```python
from build123d import *

# Parameters (mm, degrees)
EXTRUSION1_DEPTH         = 3
ENL_V_MAT_EXTRU_14_REACH = 176.1
ESQUISSE8_R              = 2
ESQUISSE10_R             = 2
ENL_V_MAT_EXTRU_16_DEPTH = 175.099861741
ENL_V_MAT_EXTRU_17_DEPTH = 175.099861741
ENL_V_MAT_EXTRU_18_DEPTH = 167.529952384
CONG_1_R                 = 3


with BuildPart() as part:
    # Esquisse1 → Extrusion1 (new body)
    with BuildSketch(Plane(origin=(0, 0, 0), x_dir=(1, 0, 0), z_dir=(0, 1, 0))):
        Polygon((-64.179491924, 79.940798285), (98.820508076, 79.940798285), (103.820508076, 74.940798285), (103.820508076, 24.940798285), (101.320508076, 15.610671266), (19.820508076, -125.551469551), (12.990381057, -127.38159657), (-30.310889132, -102.38159657), (-37.141016151, -95.551469551), (-118.641016151, 45.610671266), (-116.810889132, 52.440798285), (-73.509618943, 77.440798285), align=None)
    extrude(amount=EXTRUSION1_DEPTH)

    # Esquisse8 → Enlèv. mat.-Extru.14 (cut, up to next)
    with BuildSketch(Plane(origin=(0, 3, 0), x_dir=(1, 0, 0), z_dir=(0, 1, 0)), mode=Mode.PRIVATE) as enl_v_mat_extru_14_sk1:
        with Locations(Location((-100.570508076, 34.31163316, 0), (0, 0, 270))):
            Circle(ESQUISSE8_R)
    enl_v_mat_extru_14_tool1 = extrude(enl_v_mat_extru_14_sk1.sketch, amount=-ENL_V_MAT_EXTRU_14_REACH, mode=Mode.PRIVATE) & part.part
    # Esquisse8 → Enlèv. mat.-Extru.14 (cut, up to next)
    with BuildSketch(Plane(origin=(0, 3, 0), x_dir=(1, 0, 0), z_dir=(0, 1, 0)), mode=Mode.PRIVATE) as enl_v_mat_extru_14_sk2:
        with Locations(Location((80, 69.940798285, 0), (0, 0, 270))):
            Circle(ESQUISSE8_R)
    enl_v_mat_extru_14_tool2 = extrude(enl_v_mat_extru_14_sk2.sketch, amount=-ENL_V_MAT_EXTRU_14_REACH, mode=Mode.PRIVATE) & part.part
    # Esquisse8 → Enlèv. mat.-Extru.14 (cut, up to next)
    with BuildSketch(Plane(origin=(0, 3, 0), x_dir=(1, 0, 0), z_dir=(0, 1, 0)), mode=Mode.PRIVATE) as enl_v_mat_extru_14_sk3:
        with Locations(Location((50, 69.940798285, 0), (0, 0, 270))):
            Circle(ESQUISSE8_R)
    enl_v_mat_extru_14_tool3 = extrude(enl_v_mat_extru_14_sk3.sketch, amount=-ENL_V_MAT_EXTRU_14_REACH, mode=Mode.PRIVATE) & part.part
    # Esquisse8 → Enlèv. mat.-Extru.14 (cut, up to next)
    with BuildSketch(Plane(origin=(0, 3, 0), x_dir=(1, 0, 0), z_dir=(0, 1, 0)), mode=Mode.PRIVATE) as enl_v_mat_extru_14_sk4:
        with Locations(Location((-50.570508076, -52.290907218, 0), (0, 0, 270))):
            Circle(ESQUISSE8_R)
    enl_v_mat_extru_14_tool4 = extrude(enl_v_mat_extru_14_sk4.sketch, amount=-ENL_V_MAT_EXTRU_14_REACH, mode=Mode.PRIVATE) & part.part
    # Esquisse8 → Enlèv. mat.-Extru.14 (cut, up to next)
    with BuildSketch(Plane(origin=(0, 3, 0), x_dir=(1, 0, 0), z_dir=(0, 1, 0)), mode=Mode.PRIVATE) as enl_v_mat_extru_14_sk5:
        with Locations(Location((-35.570508076, -78.271669332, 0), (0, 0, 270))):
            Circle(ESQUISSE8_R)
    enl_v_mat_extru_14_tool5 = extrude(enl_v_mat_extru_14_sk5.sketch, amount=-ENL_V_MAT_EXTRU_14_REACH, mode=Mode.PRIVATE) & part.part
    # Esquisse8 → Enlèv. mat.-Extru.14 (cut, up to next)
    with BuildSketch(Plane(origin=(0, 3, 0), x_dir=(1, 0, 0), z_dir=(0, 1, 0)), mode=Mode.PRIVATE) as enl_v_mat_extru_14_sk6:
        with Locations(Location((-20, 69.940798285, 0), (0, 0, 270))):
            Circle(ESQUISSE8_R)
    enl_v_mat_extru_14_tool6 = extrude(enl_v_mat_extru_14_sk6.sketch, amount=-ENL_V_MAT_EXTRU_14_REACH, mode=Mode.PRIVATE) & part.part
    # Esquisse8 → Enlèv. mat.-Extru.14 (cut, up to next)
    with BuildSketch(Plane(origin=(0, 3, 0), x_dir=(1, 0, 0), z_dir=(0, 1, 0)), mode=Mode.PRIVATE) as enl_v_mat_extru_14_sk7:
        with Locations(Location((-50, 69.940798285, 0), (0, 0, 270))):
            Circle(ESQUISSE8_R)
    enl_v_mat_extru_14_tool7 = extrude(enl_v_mat_extru_14_sk7.sketch, amount=-ENL_V_MAT_EXTRU_14_REACH, mode=Mode.PRIVATE) & part.part
    # Esquisse8 → Enlèv. mat.-Extru.14 (cut, up to next)
    with BuildSketch(Plane(origin=(0, 3, 0), x_dir=(1, 0, 0), z_dir=(0, 1, 0)), mode=Mode.PRIVATE) as enl_v_mat_extru_14_sk8:
        with Locations(Location((20.570508076, -104.252431445, 0), (0, 0, 270))):
            Circle(ESQUISSE8_R)
    enl_v_mat_extru_14_tool8 = extrude(enl_v_mat_extru_14_sk8.sketch, amount=-ENL_V_MAT_EXTRU_14_REACH, mode=Mode.PRIVATE) & part.part
    # Esquisse8 → Enlèv. mat.-Extru.14 (cut, up to next)
    with BuildSketch(Plane(origin=(0, 3, 0), x_dir=(1, 0, 0), z_dir=(0, 1, 0)), mode=Mode.PRIVATE) as enl_v_mat_extru_14_sk9:
        with Locations(Location((35.570508076, -78.271669332, 0), (0, 0, 270))):
            Circle(ESQUISSE8_R)
    enl_v_mat_extru_14_tool9 = extrude(enl_v_mat_extru_14_sk9.sketch, amount=-ENL_V_MAT_EXTRU_14_REACH, mode=Mode.PRIVATE) & part.part
    # Esquisse8 → Enlèv. mat.-Extru.14 (cut, up to next)
    with BuildSketch(Plane(origin=(0, 3, 0), x_dir=(1, 0, 0), z_dir=(0, 1, 0)), mode=Mode.PRIVATE) as enl_v_mat_extru_14_sk10:
        with Locations(Location((-85.570508076, 8.330871047, 0), (0, 0, 270))):
            Circle(ESQUISSE8_R)
    enl_v_mat_extru_14_tool10 = extrude(enl_v_mat_extru_14_sk10.sketch, amount=-ENL_V_MAT_EXTRU_14_REACH, mode=Mode.PRIVATE) & part.part
    # Esquisse8 → Enlèv. mat.-Extru.14 (cut, up to next)
    with BuildSketch(Plane(origin=(0, 3, 0), x_dir=(1, 0, 0), z_dir=(0, 1, 0)), mode=Mode.PRIVATE) as enl_v_mat_extru_14_sk11:
        with Locations(Location((70.570508076, -17.649891067, 0), (0, 0, 270))):
            Circle(ESQUISSE8_R)
    enl_v_mat_extru_14_tool11 = extrude(enl_v_mat_extru_14_sk11.sketch, amount=-ENL_V_MAT_EXTRU_14_REACH, mode=Mode.PRIVATE) & part.part
    # Esquisse8 → Enlèv. mat.-Extru.14 (cut, up to next)
    with BuildSketch(Plane(origin=(0, 3, 0), x_dir=(1, 0, 0), z_dir=(0, 1, 0)), mode=Mode.PRIVATE) as enl_v_mat_extru_14_sk12:
        with Locations(Location((85.570508076, 8.330871047, 0), (0, 0, 270))):
            Circle(ESQUISSE8_R)
    enl_v_mat_extru_14_tool12 = extrude(enl_v_mat_extru_14_sk12.sketch, amount=-ENL_V_MAT_EXTRU_14_REACH, mode=Mode.PRIVATE) & part.part
    add(enl_v_mat_extru_14_tool1.solids().sort_by_distance((-100.570508, 3, -34.311633))[0], mode=Mode.SUBTRACT)
    add(enl_v_mat_extru_14_tool2.solids().sort_by_distance((80, 3, -69.940798))[0], mode=Mode.SUBTRACT)
    add(enl_v_mat_extru_14_tool3.solids().sort_by_distance((50, 3, -69.940798))[0], mode=Mode.SUBTRACT)
    add(enl_v_mat_extru_14_tool4.solids().sort_by_distance((-50.570508, 3, 52.290907))[0], mode=Mode.SUBTRACT)
    add(enl_v_mat_extru_14_tool5.solids().sort_by_distance((-35.570508, 3, 78.271669))[0], mode=Mode.SUBTRACT)
    add(enl_v_mat_extru_14_tool6.solids().sort_by_distance((-20, 3, -69.940798))[0], mode=Mode.SUBTRACT)
    add(enl_v_mat_extru_14_tool7.solids().sort_by_distance((-50, 3, -69.940798))[0], mode=Mode.SUBTRACT)
    add(enl_v_mat_extru_14_tool8.solids().sort_by_distance((20.570508, 3, 104.252431))[0], mode=Mode.SUBTRACT)
    add(enl_v_mat_extru_14_tool9.solids().sort_by_distance((35.570508, 3, 78.271669))[0], mode=Mode.SUBTRACT)
    add(enl_v_mat_extru_14_tool10.solids().sort_by_distance((-85.570508, 3, -8.330871))[0], mode=Mode.SUBTRACT)
    add(enl_v_mat_extru_14_tool11.solids().sort_by_distance((70.570508, 3, 17.649891))[0], mode=Mode.SUBTRACT)
    add(enl_v_mat_extru_14_tool12.solids().sort_by_distance((85.570508, 3, -8.330871))[0], mode=Mode.SUBTRACT)

    # Esquisse10 → Enlèv. mat.-Extru.16 (cut, through all)
    with BuildSketch(Plane(origin=(0, 3, 0), x_dir=(1, 0, 0), z_dir=(0, 1, 0))):
        with Locations(Location((-63.520181276, -17.020181276, 0), (0, 0, 270))):
            Circle(ESQUISSE10_R)
        with Locations(Location((17.020181276, -63.520181276, 0), (0, 0, 270))):
            Circle(ESQUISSE10_R)
        with Locations(Location((42.965884077, 15.839094213, 0), (0, 0, 270))):
            Circle(ESQUISSE10_R)
        with Locations(Location((-7.629221728, 8.965800345, 0), (0, 0, 270))):
            Circle(ESQUISSE10_R)
        with Locations(Location((-7.029145761, 55.985162408, 0), (0, 0, 270))):
            Circle(ESQUISSE10_R)
    extrude(amount=-ENL_V_MAT_EXTRU_16_DEPTH, mode=Mode.SUBTRACT)

    # Esquisse12 → Enlèv. mat.-Extru.17 (cut, through all)
    with BuildSketch(Plane(origin=(0, 3, 0), x_dir=(1, 0, 0), z_dir=(0, 1, 0))):
        Polygon((-30.310889132, -102.38159657), (12.990381057, -127.38159657), (19.820508076, -125.551469551), (101.320508076, 15.610671266), (103.820508076, 24.940798285), (103.820508076, 74.940798285), (98.820508076, 79.940798285), (-64.179491924, 79.940798285), (-73.509618943, 77.440798285), (-116.810889132, 52.440798285), (-118.641016151, 45.610671266), (-37.141016151, -95.551469551), align=None)
        Polygon((99.62141135, 18.66774941), (19.722431865, -119.721342532), (12.794228635, -115.721342532), (9.294228635, -121.783520358), (-28.810889132, -99.783520358), (-28.310889132, -98.917494954), (-33.444863728, -95.953393339), (-33.643960454, -95.608547695), (-113.54293994, 42.780544247), (-106.61473671, 46.780544247), (-110.11473671, 52.842722074), (-72.009618943, 74.842722074), (-71.509618943, 73.97669667), (-66.375644347, 76.940798285), (-65.977450895, 76.940798285), (93.820508076, 76.940798285), (93.820508076, 68.940798285), (100.820508076, 68.940798285), (100.820508076, 24.940798285), (99.820508076, 24.940798285), (99.820508076, 19.012595055), align=None, mode=Mode.SUBTRACT)
    extrude(amount=-ENL_V_MAT_EXTRU_17_DEPTH, mode=Mode.SUBTRACT)

    # Esquisse13 → Enlèv. mat.-Extru.18 (cut, through all)
    with BuildSketch(Plane(origin=(0, 3, 0), x_dir=(1, 0, 0), z_dir=(0, 1, 0))):
        Polygon((-70.131397208, -11.47114317), (-45.131397208, 31.830127019), (-53.791651246, 36.830127019), (-78.791651246, -6.47114317), align=None)
        Polygon((-51.291651246, 41.160254038), (-36.291651246, 67.141016151), (-27.631397208, 62.141016151), (-42.631397208, 36.160254038), align=None)
        Polygon((32.631397208, -53.480762114), (62.631397208, -1.519237886), (71.291651246, -6.519237886), (41.291651246, -58.480762114), align=None)
        Polygon((70.801270189, 22.631397208), (36.160254038, 42.631397208), (41.160254038, 51.291651246), (45.803878216, 48.610653577), (45.803878216, 65.342402688), (64.803878216, 65.342402688), (64.803878216, 46.342402688), (64.803878216, 37.640998462), (75.801270189, 31.291651246), align=None)
        Polygon((2.810889132, -65.131397208), (-36.160254038, -42.631397208), (-41.160254038, -51.291651246), (-2.189110868, -73.791651246), align=None)
    extrude(amount=-ENL_V_MAT_EXTRU_18_DEPTH, mode=Mode.SUBTRACT)

    # Congé1
    cong_1_edges = [part.edges().sort_by_distance(p)[0] for p in [
        (-70.131397208, 1.5, 11.47114317),
        (-78.791651246, 1.5, 6.47114317),
        (-53.791651246, 1.5, -36.830127019),
        (-45.131397208, 1.5, -31.830127019),
        (2.810889132, 1.5, 65.131397208),
        (-2.189110868, 1.5, 73.791651246),
        (-41.160254038, 1.5, 51.291651246),
        (-36.160254038, 1.5, 42.631397208),
        (75.801270189, 1.5, -31.291651246),
        (70.801270189, 1.5, -22.631397208),
        (36.160254038, 1.5, -42.631397208),
        (41.160254038, 1.5, -51.291651246),
        (71.291651246, 1.5, 6.519237886),
        (41.291651246, 1.5, 58.480762114),
        (32.631397208, 1.5, 53.480762114),
        (62.631397208, 1.5, 1.519237886),
        (-42.631397208, 1.5, -36.160254038),
        (-51.291651246, 1.5, -41.160254038),
        (-36.291651246, 1.5, -67.141016151),
        (-27.631397208, 1.5, -62.141016151),
    ]]
    fillet(cong_1_edges, radius=CONG_1_R)


solid = part.part
```
Model file for the job. Use its own axes, mm. A direction names the side the tool comes from. Give positions to 0.01 mm unless a question says otherwise; leave off trailing zeros. Order: outer loops, then holes, each group sorted by start corner. A loop starts at its lowest first (then second) coordinate and runs counter-clockwise, first axis right, second up.
1) Saw through at C-C, the plane y = 2.1. Count the separate pieces of the cut face and the enclosed holes in it, then the cut area to 3 significant figures.
2) Mould opens along X. For faces 1 (the flat face through (-5, 0, -1)), 2 (the flat face through (-91.33, 1.52, -63.69)), 3 (the flat face through (68.945, 1.521, -35.25)) say: +X half, -X half, draft (parallel to the pull), parting line (faces both ways), or undercut.
3) Saw through at A-A, the plane z = 31. Write the cut outline in (x, y), then the cut area to 3 significant figures.
4) Pin check, flat tips, straight feed: pin 1 (1.1 mm diameter, centred on x = 100.5, y = 1.5, fed in from +Z); pin 2 (3.5 mm diameter, centred on x = -50, z = -69.94, fed in from +Y); pin 3 (0.9 mm diameter, centred on x = 56, y = 1, fed in from +Z); pin 4 (0.9 mm diameter, centred on y = 1, z = -72, fed in from +X). Stop position of each tip, or through.
5) Saw through at B-B, the plane x = 29.5. Write the cut outline in (y, z), then the cut area to 3 significant figures.
6) Wall check: probe 1 along Z at (x, y) = (66, 0.25); probe 2 along X at (y, z) = (0.7, 7.5); probe 3 along X at (y, z) = (0.85, 64.5). Give the ranges that are in metal, low to high.
7) 3-axis set-ups, long thin cutter, end or side, ignore diameter. For faces 4 (the flat face through (-9.49, 1.52, 110.94)), 5 (the flat face through (-35.047, 1.521, -49.296)): which of +Z, -Z, +X, -X, +Y, -Y reach the whole face in a straight line?
Computed:
1. separate pieces: 1
1. enclosed holes: 22
1. area: 25,000 mm2
2. face 1: draft
2. face 2: -X half
2. face 3: undercut
3. outline: (-70.95, 0) - (45.61, 0) - (45.61, 3) - (-70.95, 3) - close; (57.16, 0) - (70.95, 0) - (70.95, 3) - (57.16, 3) - close
3. area: 391 mm2
4. pin 1: stops at z = -24.94
4. pin 2: passes through
4. pin 3: stops at z = 57.67
4. pin 4: stops at x = 93.82
5. outline: (0, -76.94) - (3, -76.94) - (3, 102.79) - (0, 102.79) - close
5. area: 539 mm2
6. probe 1: z = -76.94 to -36.95, -25.4 to 3.46, 15.68 to 39.57
6. probe 2: x = -84.51 to -76.81, -67.84 to 59.18, 70.19 to 84.51
6. probe 3: x = -51.6 to -18.28, 1.16 to 15.28, 18.76 to 51.6
7. face 4: +Z, -X, +Y, -Y
7. face 5: +Y, -Y
